```python
from build123d import *

# Parameters (mm, degrees)
SKETCH1_W           = 152.4
SKETCH1_H           = 76.2
SKETCH1_R           = 4.1656
BOSS_EXTRUDE1_DEPTH = 3.175


with BuildPart() as part:
    # Sketch1 → Boss-Extrude1 (new body, symmetric)
    with BuildSketch(Plane.XY):
        with Locations((76.2, 38.1)):
            Rectangle(SKETCH1_W, SKETCH1_H)
        with Locations((19.05, 19.05)):
            Circle(SKETCH1_R, mode=Mode.SUBTRACT)
        with Locations((57.15, 19.05)):
            Circle(SKETCH1_R, mode=Mode.SUBTRACT)
        with Locations((95.25, 19.05)):
            Circle(SKETCH1_R, mode=Mode.SUBTRACT)
        with Locations((133.35, 19.05)):
            Circle(SKETCH1_R, mode=Mode.SUBTRACT)
        with Locations((19.05, 57.15)):
            Circle(SKETCH1_R, mode=Mode.SUBTRACT)
        with Locations((57.15, 57.15)):
            Circle(SKETCH1_R, mode=Mode.SUBTRACT)
        with Locations((95.25, 57.15)):
            Circle(SKETCH1_R, mode=Mode.SUBTRACT)
        with Locations((133.35, 57.15)):
            Circle(SKETCH1_R, mode=Mode.SUBTRACT)
    extrude(amount=BOSS_EXTRUDE1_DEPTH, both=True)


solid = part.part
```
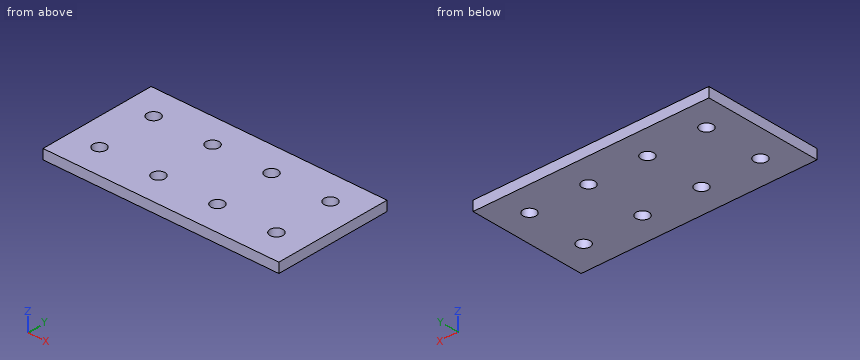
Part model, mm, in its own coordinate system. Coordinates: 2 decimals unless noted, no trailing zeros. Write each loop counter-clockwise with the first axis right and the second up, starting at its lowest first coordinate (ties: lowest second). Pieces come first, ordered by that corner, then holes.
Item 1: Slice it at D-D (y = 55.5). Write the cut outline in (x, z) (3 decimals).
Item 2: Slice it at C-C (z = 0). Count the separate pieces of the cut face and the enclosed holes in it, and give its area (3 significant figures).
Item 3: Slice it at A-A (x = 133.35). Write the cut outline in (y, z) (3 decimals).
Item 4: Probe line 1 (Y direction, x = 57.15, z = 1.75); line 2 (X direction, y = 60, z = -0.5); line 3 (X direction, y = 19, z = -1.25). List the from-to ranges inside material, lowest first.
Item 5: Slice it at B-B (y = 19.05). Write the cut outline in (x, z) (3 decimals), and give its area (3 significant figures).
Results found:
1. outline: (0, -3.175) - (15.225, -3.175) - (15.225, 3.175) - (0, 3.175) - close; (22.875, -3.175) - (53.325, -3.175) - (53.325, 3.175) - (22.875, 3.175) - close; (60.975, -3.175) - (91.425, -3.175) - (91.425, 3.175) - (60.975, 3.175) - close; (99.075, -3.175) - (129.525, -3.175) - (129.525, 3.175) - (99.075, 3.175) - close; (137.175, -3.175) - (152.4, -3.175) - (152.4, 3.175) - (137.175, 3.175) - close
2. separate pieces: 1
2. enclosed holes: 8
2. area: 11,200 mm2
3. outline: (0, -3.175) - (14.884, -3.175) - (14.884, 3.175) - (0, 3.175) - close; (23.216, -3.175) - (52.984, -3.175) - (52.984, 3.175) - (23.216, 3.175) - close; (61.316, -3.175) - (76.2, -3.175) - (76.2, 3.175) - (61.316, 3.175) - close
4. line 1: y = 0 to 14.88, 23.22 to 52.98, 61.32 to 76.2
4. line 2: x = 0 to 16.01, 22.09 to 54.11, 60.19 to 92.21, 98.29 to 130.31, 136.39 to 152.4
4. line 3: x = 0 to 14.88, 23.22 to 52.98, 61.32 to 91.08, 99.42 to 129.18, 137.52 to 152.4
5. outline: (0, -3.175) - (14.884, -3.175) - (14.884, 3.175) - (0, 3.175) - close; (23.216, -3.175) - (52.984, -3.175) - (52.984, 3.175) - (23.216, 3.175) - close; (61.316, -3.175) - (91.084, -3.175) - (91.084, 3.175) - (61.316, 3.175) - close; (99.416, -3.175) - (129.184, -3.175) - (129.184, 3.175) - (99.416, 3.175) - close; (137.516, -3.175) - (152.4, -3.175) - (152.4, 3.175) - (137.516, 3.175) - close
5. area: 756 mm2
